```python
from build123d import *

# Parameters (mm, degrees)
F1_DEPTH = 63.5
F0_W     = 25.4
F0_H     = 19.05
F2_DEPTH = 25.4
F0_H_2   = 4.7498
F0_H_3   = 4.7752
F4_DEPTH = 7.9375
F5_R     = 6.35


with BuildPart() as f1:
    # F0 (on Front) → F1 (new body, symmetric)
    with BuildSketch(Plane.XZ):
        Polygon((-41.275, 9.525), (-41.275, -9.525), (41.275, -9.525), (41.275, 9.525), (22.225, 9.525), align=None)
    extrude(amount=F1_DEPTH, both=True)

    # F0 (on Front) → F2 (join, symmetric)
    with BuildSketch(Plane.XZ):
        with BuildLine():
            Line((22.225, 9.525), (41.275, 9.525))
            Line((41.275, 9.525), (41.275, 27.0002))
            ThreePointArc((41.275, 27.0002), (45.9246798487, 38.2255201513), (57.15, 42.8752))
            Line((57.15, 42.8752), (60.325, 42.8752))
            Line((60.325, 42.8752), (60.325, 61.9252))
            Line((60.325, 61.9252), (57.15, 61.9252))
            add(Edge.make_bspline(
                [(53.8635781544, 61.7702310102), (54.9491847021, 61.8205950904), (56.0446147523, 61.8720257258), (57.15, 61.9252)],
                knots=[108.9349794531, 108.9349794531, 108.9349794531, 108.9349794531, 111.5045361635, 111.5045361635, 111.5045361635, 111.5045361635], degree=3))
            ThreePointArc((53.8635781544, 61.7702310102), (31.3184891271, 50.5052775583), (22.225, 27.0002))
            Line((22.225, 27.0002), (22.225, 9.525))
        make_face()
        with Locations((73.025, 52.4002)):
            Rectangle(F0_W, F0_H)
    extrude(amount=F2_DEPTH, both=True)

    # F0 (on Front) → F3 (revolve)
    with BuildSketch(Plane.XZ):
        with Locations((98.425, 64.3001)):
            Rectangle(F0_W, F0_H_2)
        with Locations((98.425, 40.4876)):
            Rectangle(F0_W, F0_H_3)
        with Locations((98.425, 52.4002)):
            Rectangle(F0_W, F0_H)
    revolve(axis=Axis((85.725, 0, 52.3875), (0, 0, 1)))

    # F0 (on Front) → F4 (join, symmetric)
    with BuildSketch(Plane.XZ):
        with BuildLine():
            add(Edge.make_bspline(
                [(-41.275, 9.525), (-20.5281487987, 59.4168244671), (7.8398704502, 59.6350728281), (53.8635781544, 61.7702310102)],
                knots=[0, 0, 0, 0, 108.9349794531, 108.9349794531, 108.9349794531, 108.9349794531], degree=3))
            Line((-41.275, 9.525), (22.225, 9.525))
            Line((22.225, 9.525), (22.225, 27.0002))
            ThreePointArc((22.225, 27.0002), (31.3184891271, 50.5052775583), (53.8635781544, 61.7702310102))
        make_face()
    extrude(amount=F4_DEPTH, both=True)

    # F5
    f5_edges = [f1.edges().sort_by_distance(p)[0] for p in [
        (41.275, -63.5, 0),
        (-41.275, -63.5, 0),
        (41.275, 63.5, 0),
        (-41.275, 63.5, 0),
    ]]
    fillet(f5_edges, radius=F5_R)


solid = f1.part
```
Geometry check sheet. Reference: the model listing, model coordinates, mm. A direction names the side the tool comes from. Give positions to 0.01 mm unless a question says otherwise; leave off trailing zeros. Order: outer loops, then holes, each group sorted by start corner. A loop starts at its lowest first (then second) coordinate and runs counter-clockwise, first axis right, second up. Notation, with made-up numbers: (5.5, 53) -> (56.5, 53) arc R26 cw to (56.5, 77) -> close; hole circle Ø7 at (65.5, 21.5). An arc over 180 degrees is marked (long way). Write each question's results on one line, items separated by ' | '. Start each with the question number.
(1) Access from +Z, -Z, +X, -X, +Y, -Y to the whole of each face (thin tool, end or side, straight path). Record for faces 1 (the face through (-4, -7.938, 30)), 2 (the face through (41.275, -1, 4)), 3 (the face through (60, -2, 61.925)).
(2) Scan lines: line 1 (Z direction, x = 58.5, y = -10); line 2 (Y direction, x = 39, z = 24.5); line 3 (Y direction, x = -25.5, z = 33.5). Record each from-to range of solid material in increasing order.
(3) Gauge pin test, flat ends, axial feed: P1, Ø15.5, axis at x = 39.5, z = 30, coming from the +Y side; P2, Ø1, axis at x = 7, z = 28, coming from the +Y side; P3, Ø2, axis at x = 71.5, z = 45, coming from the -Y side. Record the tip position at first contact, or that the pin passes through.
(4) Sectioned sample at A-A (y = 29.5). Enter the section's corners in (x, z) (3 decimals).
(5) Sectioned sample at B-B (x = 80). Enter the section's corners in (y, z) (3 decimals), plus the area to 3 significant figures.
Answer below:
1) face 1: +Z, -X, -Y | face 2: -Z, +X, +Y, -Y | face 3: +Z, -X
2) line 1: 42.88 to 61.93 | line 2: -25.4 to 25.4 | line 3: -7.94 to 7.94
3) P1: y = 25.4 | P2: y = 7.94 | P3: y = -25.4
4) outline: (-41.275, -9.525) -> (41.275, -9.525) -> (41.275, 9.525) -> (-41.275, 9.525) -> close
5) outline: (-25.4, 42.875) -> (-24.746, 42.875) -> (-24.746, 38.1) -> (24.746, 38.1) -> (24.746, 42.875) -> (25.4, 42.875) -> (25.4, 61.925) -> (24.746, 61.925) -> (24.746, 66.675) -> (-24.746, 66.675) -> (-24.746, 61.925) -> (-25.4, 61.925) -> close | area: 1,440 mm2
